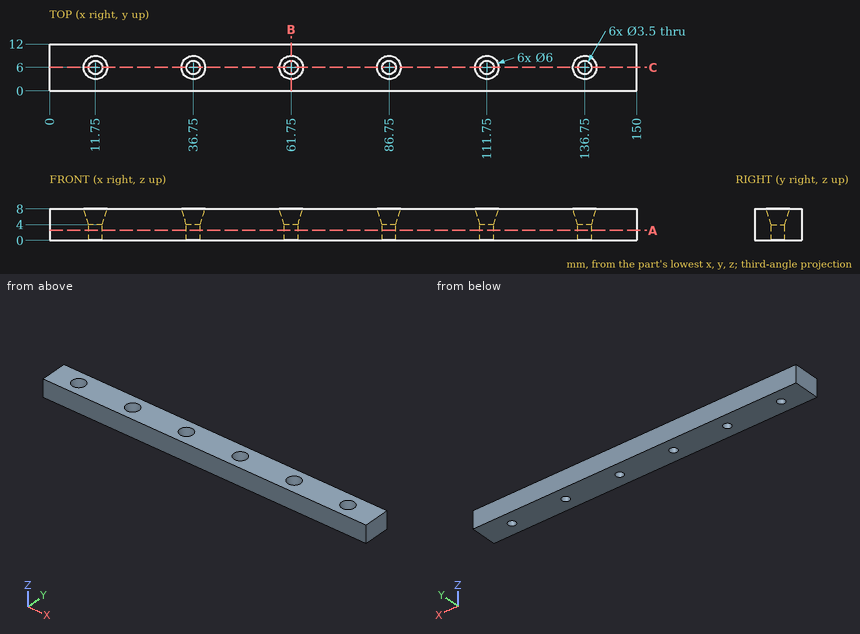
Design review of the part shown in the three views and the two pictorial views. Dimensions are in mm from the part's minimum x, y and z. Round coordinates to 2 decimals unless told otherwise and drop trailing zeros. Write each loop counter-clockwise with the first axis right and the second up, starting at its lowest first coordinate (ties: lowest second). Pieces come first, ordered by that corner, then holes.
Item 1: Consider section B-B on x = 61.75. Give the boundary of the cut face in (y, z), and give its area (3 significant figures).
Item 2: Consider section A-A on z = 2.5. Give the boundary of the cut face in (x, y).
Item 3: Consider section C-C on y = 6. Count the separate pieces of the cut face and the enclosed holes in it, and give its area (3 significant figures).
Item 4: Wall thickness on L1, parallel to Y at x = 11.75, z = 1.1: over which ranges is the line inside the solid? List them lowest first.
Check values:
1. outline: (0, 0) - (4.25, 0) - (4.25, 4) - (3, 8) - (0, 8) - close; (7.75, 0) - (12, 0) - (12, 8) - (9, 8) - (7.75, 4) - close
1. area: 63.0 mm2
2. outline: (0, 0) - (150, 0) - (150, 12) - (0, 12) - close; hole circle Ø3.5 at (11.75, 6); hole circle Ø3.5 at (36.75, 6); hole circle Ø3.5 at (61.75, 6); hole circle Ø3.5 at (86.75, 6); hole circle Ø3.5 at (111.75, 6); hole circle Ø3.5 at (136.75, 6)
3. separate pieces: 7
3. enclosed holes: 0
3. area: 1,000 mm2
4. L1: y = 0 to 4.25, 7.75 to 12
